from build123d import *

# Parameters (mm, degrees)
SKETCH1_W           = 45
SKETCH1_H           = 70
BOSS_EXTRUDE1_DEPTH = 10
SKETCH3_R           = 4.15
CUT_EXTRUDE2_DEPTH  = 11
SKETCH5_R           = 4.15
BOSS_EXTRUDE2_DEPTH = 9
CHAMFER1_SIZE       = 1
CHAMFER1_SIZE2      = 1.191753593
FILLET1_R           = 10
CUT_EXTRUDE3_DEPTH  = 20
FILLET2_R           = 8


with BuildPart() as part:
    # Sketch1 → Boss-Extrude1 (new body)
    with BuildSketch(Plane(origin=(0, 0, 0), x_dir=(1, 0, 0), z_dir=(0, 1, 0))):
        Rectangle(SKETCH1_W, SKETCH1_H)
    extrude(amount=BOSS_EXTRUDE1_DEPTH)

    # Sketch3 → Cut-Extrude2 (cut, through all)
    with BuildSketch(Plane.XZ):
        with Locations((15, 25)):
            Circle(SKETCH3_R)
        with Locations((15, -25)):
            Circle(SKETCH3_R)
        with Locations((-15, -25)):
            Circle(SKETCH3_R)
        with Locations((-15, 25)):
            Circle(SKETCH3_R)
    extrude(amount=-CUT_EXTRUDE2_DEPTH, mode=Mode.SUBTRACT)

    # Sketch5 → Boss-Extrude2 (add)
    with BuildSketch(Plane(origin=(0, 10, 0), x_dir=(1, 0, 0), z_dir=(0, 1, 0))):
        Polygon((-5.15, -35), (-22.5, -35), (-22.5, 35), (22.5, 35), (22.5, -35), (5.15, -35), (5.130229348, -34.949305848), (5.15, 31), (-5.15, 31), align=None)
        with Locations((-15, 25)):
            Circle(SKETCH5_R, mode=Mode.SUBTRACT)
        with Locations((15, 25)):
            Circle(SKETCH5_R, mode=Mode.SUBTRACT)
        with Locations((15, -25)):
            Circle(SKETCH5_R, mode=Mode.SUBTRACT)
        with Locations((-15, -25)):
            Circle(SKETCH5_R, mode=Mode.SUBTRACT)
    extrude(amount=BOSS_EXTRUDE2_DEPTH)

    # Chamfer1
    chamfer1_edges = [part.edges().sort_by_distance(p)[0] for p in [
        (-19.15, 0, -25),
        (-19.15, 0, 25),
        (10.85, 0, 25),
        (10.85, 0, -25),
    ]]
    chamfer1_side = [part.faces().sort_by_distance(p)[0] for p in [
        (0, 0, 0),
    ]]
    chamfer(chamfer1_edges, length=CHAMFER1_SIZE, length2=CHAMFER1_SIZE2, reference=chamfer1_side[0])

    # Fillet1
    fillet1_edges = [part.edges().sort_by_distance(p)[0] for p in [
        (-22.5, 9.5, -35),
        (22.5, 9.5, -35),
        (22.5, 9.5, 35),
        (-22.5, 9.5, 35),
    ]]
    fillet(fillet1_edges, radius=FILLET1_R)

    # Sketch6 → Cut-Extrude3 (cut, through all)
    with BuildSketch(Plane(origin=(0, 19, 0), x_dir=(1, 0, 0), z_dir=(0, 1, 0))):
        with BuildLine():
            Line((-12.5, 35), (12.5, 35))
            ThreePointArc((12.5, 35), (0, 33.26906369), (-12.5, 35))
        make_face()
    extrude(amount=-CUT_EXTRUDE3_DEPTH, mode=Mode.SUBTRACT)

    # Fillet2
    fillet2_edges = [part.edges().sort_by_distance(p)[0] for p in [
        (-12.5, 9.5, -35),
        (12.5, 9.5, -35),
    ]]
    fillet(fillet2_edges, radius=FILLET2_R)


solid = part.part
Check sheet for the modelled part. Datum: model origin and axes. Units: mm. A direction names the side the tool comes from. Give positions to 0.01 mm unless a question says otherwise; leave off trailing zeros. Order: outer loops, then holes, each group sorted by start corner. A loop starts at its lowest first (then second) coordinate and runs counter-clockwise, first axis right, second up. Notation, with made-up numbers: (11.5, -23) - (70.5, -23) arc R19 cw to (70.5, 6) - close; hole circle Ø4 at (48, 8). An arc over 180 degrees is marked (long way). Answer as CSV lines item,"result".
1. Tool access check on faces 1 (the face through (14.1, 9.97, 29.05)), 2 (the face through (0, 10, 2)). Record the directions out of +Z, -Z, +X, -X, +Y, -Y that give a thin tool (end or side, any length) a straight path to the whole face; none if there is none.
Result sheet:
face 1,"+Y, -Y"
face 2,"+Z, +Y"
2. Go/stop test with flat-tipped pins: P1, Ø2, axis at x = -16, y = 6.5, coming from the -Z side; P2, Ø5, axis at x = 15, z = 25, coming from the +Y side; P3, Ø4.5, axis at x = 1, y = 13.5, coming from the +Z side; P4, Ø8, axis at x = 1, z = 6, coming from the +Y side. Record where each tip stops, or that it passes through.
Result sheet:
P1,"z = -34.68"
P2,"through"
P3,"z = -31"
P4,"y = 10"
3. Section check B-B (z = -0.5). Record the boundary of the cut face in (x, y).
Result sheet:
outline,"(-22.5, 0) - (22.5, 0) - (22.5, 19) - (5.14, 19) - (5.14, 10) - (-5.15, 10) - (-5.15, 19) - (-22.5, 19) - close"
4. Mould release check, pull along X, two halves, no side actions. Record for faces 3 (the face through (5.3, 19, -0.4)), 4 (the face through (14.1, 9.97, -20.95)), 5 (the face through (20.58, 9.37, -30.89)): released by +X, released by -X, zero draft, split by the parting line, or undercut.
Result sheet:
face 3,"zero draft"
face 4,"undercut"
face 5,"released by +X"
5. Scan lines: probe 1 along X at (y, z) = (6.25, 25); probe 2 along X at (y, z) = (12, 25); probe 3 along Z at (x, y) = (-15, 13.5). Record each from-to range of solid material in increasing order. Write a range as from..to.
Result sheet:
probe 1,"-22.5..-19.15, -10.85..10.85, 19.15..22.5"
probe 2,"-22.5..-19.15, -10.85..-5.15, 5.13..10.85, 19.15..22.5"
probe 3,"-34.68..-29.15, -20.85..20.85, 29.15..34.68"
6. Section check A-A (y = 8.5). State how many separate pieces and enclosed holes the cut face has, then the cut area to 3 significant figures.
Result sheet:
separate pieces,"1"
enclosed holes,"4"
area,"2,820 mm²"
